The listing builds one solid part. Answer for the finished solid, in the listing's coordinates (mm). A direction names the side the tool comes from. Give positions to 0.01 mm unless a question says otherwise; leave off trailing zeros. Write each loop counter-clockwise with the first axis right and the second up, starting at its lowest first coordinate (ties: lowest second). Pieces come first, ordered by that corner, then holes. Notation, with made-up numbers: (14.5, -22) -> (35.5, -22) arc R30 cw to (35.5, 4) -> close; hole circle Ø10 at (17, 60.5). An arc over 180 degrees is marked (long way). Use CSV: the item, a comma, the result in double quotes. Start each with the question number.
from build123d import *

# Parameters (mm, degrees)
SKETCH1_R           = 2.75
BOSS_EXTRUDE1_DEPTH = 7
SKETCH2_R           = 2.75
SKETCH2_R_2         = 1.75
BOSS_EXTRUDE2_DEPTH = 2


with BuildPart() as part:
    # Sketch1 → Boss-Extrude1 (new body)
    with BuildSketch(Plane(origin=(0, 0, 0), x_dir=(1, 0, 0), z_dir=(0, 1, 0))):
        with BuildLine():
            ThreePointArc((-1.04, 4.890644129), (-1.545084972, 4.755282581), (-2.033270819, 4.567910876))
            ThreePointArc((-2.033270819, 4.567910876), (-2.996312027, 5.563972943), (-4.181105534, 6.282201566))
            Line((-4.181105534, 6.282201566), (-4.682696071, 5.917774709))
            ThreePointArc((-4.682696071, 5.917774709), (-4.365741387, 4.569024274), (-3.716026168, 3.345317552))
            ThreePointArc((-3.716026168, 3.345317552), (-4.045084972, 2.938926261), (-4.329901294, 2.500390926))
            ThreePointArc((-4.329901294, 2.500390926), (-5.69448859, 2.740160647), (-7.075170865, 2.624815658))
            Line((-7.075170865, 2.624815658), (-7.266761401, 2.035160618))
            ThreePointArc((-7.266761401, 2.035160618), (-6.217564061, 1.130299882), (-4.972656642, 0.522193372))
            ThreePointArc((-4.972656642, 0.522193372), (-5, 0), (-4.972656642, -0.522193372))
            ThreePointArc((-4.972656642, -0.522193372), (-6.217564061, -1.130299882), (-7.266761401, -2.035160618))
            Line((-7.266761401, -2.035160618), (-7.075170865, -2.624815658))
            ThreePointArc((-7.075170865, -2.624815658), (-5.69448859, -2.740160647), (-4.329901294, -2.500390926))
            ThreePointArc((-4.329901294, -2.500390926), (-4.045084972, -2.938926261), (-3.716026168, -3.345317552))
            ThreePointArc((-3.716026168, -3.345317552), (-4.365741387, -4.569024274), (-4.682696071, -5.917774709))
            Line((-4.682696071, -5.917774709), (-4.181105534, -6.282201566))
            ThreePointArc((-4.181105534, -6.282201566), (-2.996312027, -5.563972943), (-2.033270819, -4.567910876))
            ThreePointArc((-2.033270819, -4.567910876), (-1.545084972, -4.755282581), (-1.04, -4.890644129))
            ThreePointArc((-1.04, -4.890644129), (-0.84635389, -6.262536688), (-0.31, -7.54))
            Line((-0.31, -7.54), (0.31, -7.54))
            ThreePointArc((0.31, -7.54), (0.84635389, -6.262536688), (1.04, -4.890644129))
            ThreePointArc((1.04, -4.890644129), (1.545084972, -4.755282581), (2.033270819, -4.567910876))
            ThreePointArc((2.033270819, -4.567910876), (2.996312027, -5.563972943), (4.181105534, -6.282201566))
            Line((4.181105534, -6.282201566), (4.682696071, -5.917774709))
            ThreePointArc((4.682696071, -5.917774709), (4.365741387, -4.569024274), (3.716026168, -3.345317552))
            ThreePointArc((3.716026168, -3.345317552), (4.045084972, -2.938926261), (4.329901294, -2.500390926))
            ThreePointArc((4.329901294, -2.500390926), (5.69448859, -2.740160647), (7.075170865, -2.624815658))
            Line((7.075170865, -2.624815658), (7.266761401, -2.035160618))
            ThreePointArc((7.266761401, -2.035160618), (6.217564061, -1.130299882), (4.972656642, -0.522193372))
            ThreePointArc((4.972656642, -0.522193372), (5, 0), (4.972656642, 0.522193372))
            ThreePointArc((4.972656642, 0.522193372), (6.217564061, 1.130299882), (7.266761401, 2.035160618))
            Line((7.266761401, 2.035160618), (7.075170865, 2.624815658))
            ThreePointArc((7.075170865, 2.624815658), (5.69448859, 2.740160647), (4.329901294, 2.500390926))
            ThreePointArc((4.329901294, 2.500390926), (4.045084972, 2.938926261), (3.716026168, 3.345317552))
            ThreePointArc((3.716026168, 3.345317552), (4.365741387, 4.569024274), (4.682696071, 5.917774709))
            Line((4.682696071, 5.917774709), (4.181105534, 6.282201566))
            ThreePointArc((4.181105534, 6.282201566), (2.996312027, 5.563972943), (2.033270819, 4.567910876))
            ThreePointArc((2.033270819, 4.567910876), (1.545084972, 4.755282581), (1.04, 4.890644129))
            ThreePointArc((1.04, 4.890644129), (0.84635389, 6.262536688), (0.31, 7.54))
            Line((0.31, 7.54), (-0.31, 7.54))
            ThreePointArc((-0.31, 7.54), (-0.84635389, 6.262536688), (-1.04, 4.890644129))
        make_face()
        with Locations(Location((0, 0, 0), (0, 0, 270))):
            Circle(SKETCH1_R, mode=Mode.SUBTRACT)
    extrude(amount=BOSS_EXTRUDE1_DEPTH)

    # Sketch2 → Boss-Extrude2 (add)
    with BuildSketch(Plane.XZ):
        with Locations(Location((0, 0, 0), (0, 0, 270))):
            Circle(SKETCH2_R)
        with Locations(Location((0, 0, 0), (0, 0, 270))):
            Circle(SKETCH2_R_2, mode=Mode.SUBTRACT)
    extrude(amount=-BOSS_EXTRUDE2_DEPTH)


solid = part.part
Q1. Flat-ended cylindrical pins translate along their axes: pin 1 Ø1 at (x, z) = (-1, 0) entering from +Y (3 decimals); pin 2 Ø1.5 at (x, y) = (3, 2.5) entering from +Z; pin 3 Ø3 at (y, z) = (2.5, 1) entering from +X; pin 4 Ø1.5 at (y, z) = (4, -5) entering from -X. Find the tip coordinate at first contact, or state that the pin passes through.
Q2. Section B-B on z = 0 is taken. Give the vertices of the cut face in (x, y).
Q3. Section D-D on z = -4 is taken. Give the vertices of the cut face in (x, y).
Q4. Section C-C on z = 2.25 is taken. Give the vertices of the cut face in (x, y).
Q5. Section A-A on x = 0 is taken. Give the vertices of the cut face in (y, z), then the cut area to 3 significant figures.
Q6. Straight lines are drawn through the part: L1, parallel to X at y = 3.5, z = 0; L2, parallel to Z at x = -3.5, y = 5.25; L3, parallel to X at y = 1.1, z = 0. For each, find the intervals that lie inside material, in ascending order.
Q7. For faces 5 (the face through (-2.685, 4.465, -0.596)), 6 (the face through (1.552, 3.451, -4.753)), 7 (the face through (-4.36, 3.45, 4.55)), 8 (the face through (1.538, 3.451, 4.758)), 9 (the face through (6.2, 3.45, -1.12)), determine the directions among +Z, -Z, +X, -X, +Y, -Y from which every point of the face is accessible in a straight line to the end or side of a thin tool.
Q8. The mould has two halves that part along Z. Classify faces 1 (the face through (0.84, 3.45, 6.28)), 2 (the face through (0.851, 3.451, -6.244)), 3 (the face through (4, 3, 3)), 4 (the face through (4.373, 3.451, 4.587)): +Z half, -Z half, draft (parallel to the pull), parting line (faces both ways), or undercut.
Output:
1,pin 1,"through"
1,pin 2,"z = 6.07"
1,pin 3,"x = 7.27"
1,pin 4,"x = -4.66"
2,outline,"(-5, 0) -> (-1.75, 0) -> (-1.75, 2) -> (-2.75, 2) -> (-2.75, 7) -> (-5, 7) -> close; (1.75, 0) -> (5, 0) -> (5, 7) -> (2.75, 7) -> (2.75, 2) -> (1.75, 2) -> close"
3,outline,"(-4.11, 0) -> (4.11, 0) -> (4.11, 7) -> (-4.11, 7) -> close"
4,outline,"(-7.2, 0) -> (7.2, 0) -> (7.2, 7) -> (1.58, 7) -> (1.58, 2) -> (-1.58, 2) -> (-1.58, 7) -> (-7.2, 7) -> close"
5,outline,"(0, -7.54) -> (7, -7.54) -> (7, -2.75) -> (2, -2.75) -> (2, -1.75) -> (0, -1.75) -> close; (0, 1.75) -> (2, 1.75) -> (2, 2.75) -> (7, 2.75) -> (7, 7.54) -> (0, 7.54) -> close"
5,area,"71.1 mm²"
6,L1,"-5 to -2.75, 2.75 to 5"
6,L2,"-5.92 to 5.92"
6,L3,"-5 to -1.75, 1.75 to 5"
7,face 5,"+Y"
7,face 6,"-Z, +Y, -Y"
7,face 7,"-X, +Y, -Y"
7,face 8,"+Z, +Y, -Y"
7,face 9,"+X, +Y, -Y"
8,face 1,"+Z half"
8,face 2,"-Z half"
8,face 3,"undercut"
8,face 4,"undercut"
